For this review, take the finished solid that the model builds, in its own axes (mm). Face numbers are marked on the shaded views. Round coordinates to 2 decimals unless told otherwise and drop trailing zeros. Write each loop counter-clockwise with the first axis right and the second up, starting at its lowest first coordinate (ties: lowest second). Pieces come first, ordered by that corner, then holes. Notation, with made-up numbers: (16.25, 38.5) -> (75.25, 38.5) arc R15 ccw to (75.25, 53.5) -> close; hole circle Ø10 at (67, 49.25). An arc over 180 degrees is marked (long way). Answer in a Markdown table with one row per item.
Autodesk Inventor part; units mm, degrees
ref_plane "YZ Plane" through (0, 0, 0) normal (1, 0, 0) x (0, 1, 0)
ref_plane "XZ Plane" through (0, 0, 0) normal (0, 1, 0) x (-1, 0, 0)
ref_plane "XY Plane" through (0, 0, 0) normal (0, 0, 1) x (1, 0, 0)
sketch "Szkic8" plane through (0, 0, 0) normal (0, 1, 0) x (-1, 0, 0)
  circle A0 centre (0, 0) radius 38.05
  circle A1 centre (0, 0) radius 36.45
  dimension "d53" = 76.1
  dimension "d54" = 1.6
extrude "Wyciągnięcie proste2" add sketch "Szkic8" along normal mid plane 268
sketch "Szkic13" plane through (0, 0, 0) normal (0, 0, 1) x (1, 0, 0)
  circle A0 centre (0, 0) radius 12.7
  circle A1 centre (0, 0) radius 11.1
  dimension "d67" = 25.4
  dimension "d68" = 1.6
extrude "Wyciągnięcie proste6" add sketch "Szkic13" along normal blind 41
sketch "Szkic14" plane through (0, 0, 41) normal (0, 0, 1) x (1, 0, 0)
  circle A0 centre (0, 0) radius 11.1
extrude "Wyciągnięcie proste7" cut sketch "Szkic14" against normal blind 41
sketch "Szkic15" plane through (0, -134, 0) normal (0, -1, 0) x (1, 0, 0)
  circle A0 centre (0, 0) radius 36.45
extrude "Wyciągnięcie proste8" cut sketch "Szkic15" against normal blind 268
fillet "Zaokrąglenie3" radius 1.6 2 edges at (-0.0006, 12.7, 38.05) (-0.0007, -12.7, 38.05)
fillet "Zaokrąglenie4" radius 3.2 2 edges at (0.0022, -11.1, 36.45) (0, 11.1, 36.45)
equation "\"d53\" = OD"
equation "\"d54\" = THK"
equation "\"d55\" = L1"
equation "\"d67\" = OD2"
equation "\"d68\" = THK"
equation "\"d69\" = L2"
equation "\"d71\" = L2"
equation "\"d73\" = L1"
equation "\"d75\" = THK"
equation "\"d76\" = 2 * THK"
equation "\"SzerokośćGięciaPodcięcia\" = Grubość"
equation "\"RozmiarPodcięciaNarożnika\" = 4 * Grubość"
equation "\"PromieńPrzejścia\" = PromieńGięcia"
equation "\"Rozmiar_promienia_Jacobiego\" = PromieńGięcia"
equation "\"Wielk_odstępu\" = Grubość"
equation "\"d2\" = PromieńGięcia"
equation "\"d23\" = PromieńGięcia"
equation "\"OD\" = 76.1"
equation "\"THK\" = 1.6"
equation "\"L1\" = 268"
equation "\"L2\" = 41"
equation "\"OD2\" = 25.4"
properties part number "Trójnik red. krótki  Ø76,1 25,4 76,1 s=1,6 L=268" material "304"
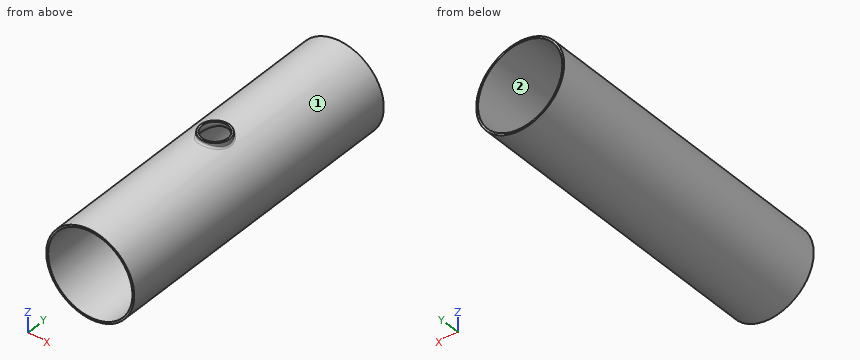
1) Mouldability with a two-part tool opening along X and no side actions: class the marked faces 1 and 2 as pulls with the +X half, pulls with the -X half, needs draft (parallel to the pull), parting line crosses it, or undercut.
Solved:
| item | result |
|---|---|
| face 1 | parting line crosses it |
| face 2 | undercut |
2) Consider section D-D on x = 0. State how many separate pieces and enclosed holes the cut face has, then the cut area to 3 significant figures.
Solved:
| item | result |
|---|---|
| separate pieces | 3 |
| enclosed holes | 0 |
| area | 828 mm² |
3) Consider section A-A on z = 0. State the section outline as (x, y) points, then the cut area to 3 significant figures.
Solved:
| item | result |
|---|---|
| outline | (-38.05, -134) -> (-36.45, -134) -> (-36.45, 134) -> (-38.05, 134) -> close; (36.45, -134) -> (38.05, -134) -> (38.05, 134) -> (36.45, 134) -> close |
| area | 858 mm² |
4) For line 1 (X direction, y = 0, z = 40.2); line 2 (Z direction, x = 0, y = 67); line 3 (Z direction, x = -13.5, y = -45.5), list the stretches that pass through material, from the lowest coordinate up. Write a range as [from, to].
Solved:
| item | result |
|---|---|
| line 1 | [-12.7, -11.1], [11.1, 12.7] |
| line 2 | [-38.05, -36.45], [36.45, 38.05] |
| line 3 | [-35.57, -33.86], [33.86, 35.57] |
5) Consider section B-B on x = -21.5. State the section outline as (y, z) points, then the cut area to 3 significant figures.
Solved:
| item | result |
|---|---|
| outline | (-134, -31.39) -> (134, -31.39) -> (134, -29.43) -> (-134, -29.43) -> close; (-134, 29.43) -> (134, 29.43) -> (134, 31.39) -> (-134, 31.39) -> close |
| area | 1,050 mm² |
6) Clearance check with flat-ended pins moving along their axes: pin 1 Ø4 at (y, z) = (-23, 18.5) entering from -X; pin 2 Ø2 at (x, y) = (-18.5, 83) entering from -Z; pin 3 Ø4 at (y, z) = (-57, 18) entering from -X. State where each tip first meets the part, or that it passes through.
Solved:
| item | result |
|---|---|
| pin 1 | x = -34.29 |
| pin 2 | z = -33.79 |
| pin 3 | x = -34.52 |
7) Consider section C-C on y = -83.5. State the section outline as (x, z) points.
Solved:
| item | result |
|---|---|
| outline | circle Ø76.1 at (0, 0); hole circle Ø72.9 at (0, 0) |
